Geometry: final body of the model. Coordinates: model frame, mm. A direction names the side the tool comes from. Round coordinates to 2 decimals unless told otherwise and drop trailing zeros. Loops run counter-clockwise (first coordinate to the right, second up) from the corner with the lowest first, then second, coordinate; pieces in that order, holes last. Notation, with made-up numbers: M -37.5,74 L -0.5,74 A12 cw -0.5,93 Z; hole C 0.25,87.5 d10. An arc over 180 degrees is marked long. Return JSON: item names as keys, results as strings.
from build123d import *

# Parameters (mm, degrees)
SKETCH1_R               = 6.35
BASE_BODY_DEPTH         = 10
SKETCH2_R               = 2.1
SHAFT_BEARING_CUT_DEPTH = 11
SKETCH3_OUTSIDE_W       = 18.812
SKETCH3_OUTSIDE_H       = 18.812
SKETCH3_OUTSIDE_R       = 4.1
LATHE_CUT_DEPTH         = 7.3


with BuildPart() as part:
    # Sketch1 → base_body (new body)
    with BuildSketch(Plane(origin=(0, 0, 0), x_dir=(1, 0, 0), z_dir=(0, 1, 0))):
        Circle(SKETCH1_R)
    extrude(amount=BASE_BODY_DEPTH)

    # Sketch2 → shaft_bearing_cut (cut, through all)
    with BuildSketch(Plane(origin=(0, 10, 0), x_dir=(1, 0, 0), z_dir=(0, 1, 0))):
        Circle(SKETCH2_R)
    extrude(amount=-SHAFT_BEARING_CUT_DEPTH, mode=Mode.SUBTRACT)

    # Sketch3 outside → lathe_cut (cut)
    with BuildSketch(Plane(origin=(0, 10, 0), x_dir=(1, 0, 0), z_dir=(0, 1, 0))):
        Rectangle(SKETCH3_OUTSIDE_W, SKETCH3_OUTSIDE_H)
        Circle(SKETCH3_OUTSIDE_R, mode=Mode.SUBTRACT)
    extrude(amount=-LATHE_CUT_DEPTH, mode=Mode.SUBTRACT)


solid = part.part
Q1. Section query D-D (x = -2.5). Output: boundary loops of the cut face in (y, z), plus the area to 3 significant figures.
Determined:
{"outline": "M 0,-5.84 L 2.7,-5.84 L 2.7,-3.25 L 10,-3.25 L 10,3.25 L 2.7,3.25 L 2.7,5.84 L 0,5.84 Z", "area": "79.0 mm^2"}
Q2. Section query B-B (z = 0). Output: boundary loops of the cut face in (x, y).
Determined:
{"outline": "M -6.35,0 L -2.1,0 L -2.1,10 L -4.1,10 L -4.1,2.7 L -6.35,2.7 Z; M 2.1,0 L 6.35,0 L 6.35,2.7 L 4.1,2.7 L 4.1,10 L 2.1,10 Z"}
Q3. Section query A-A (x = 0). Output: boundary loops of the cut face in (y, z).
Determined:
{"outline": "M 0,-6.35 L 2.7,-6.35 L 2.7,-4.1 L 10,-4.1 L 10,-2.1 L 0,-2.1 Z; M 0,2.1 L 10,2.1 L 10,4.1 L 2.7,4.1 L 2.7,6.35 L 0,6.35 Z"}
Q4. Material intervals for L1, parallel to X at y = 3.5, z = 0; L2, parallel to Y at x = 1, z = -4.25, sorted ascending.
Determined:
{"L1": "x = -4.1 to -2.1, 2.1 to 4.1", "L2": "y = 0 to 2.7"}
Q5. Reachability of faces 1 (the flat face through (1.3, 2.7, 4.1)), 2 (the flat face through (-2, 0, -2)) from +Z, -Z, +X, -X, +Y, -Y: full face, straight path, thin tool, end or side. Return the list, or none.
Determined:
{"face 1": "+Y", "face 2": "+Z, -Z, +X, -X, -Y"}
Q6. Pin query (flat end, axial travel): pin 1 (5 mm diameter, centred on x = 2.5, y = 5.5, fed in from -Z); pin 2 (1 mm diameter, centred on x = -2.5, z = 1, fed in from -Y); pin 3 (6 mm diameter, centred on x = -4.5, y = 3.5, fed in from -Z); pin 4 (6 mm diameter, centred on x = -4, y = 7.5, fed in from -Z). Return the tip coordinate at first contact, or that it passes through.
Determined:
{"pin 1": "stops at z = -4.1", "pin 2": "stops at y = 0", "pin 3": "stops at z = -6.14", "pin 4": "stops at z = -3.98"}
Q7. Section query C-C (y = 1.25). Output: boundary loops of the cut face in (x, z), plus the area to 3 significant figures.
Determined:
{"outline": "C 0,0 d12.7; hole C 0,0 d4.2", "area": "113 mm^2"}
Q8. Pull-direction query (Z, two-part tool) for faces 3 (the cylindrical face through (-0.534, 6.401, -4.065)), 4 (the flat face through (2, 10, 2)), 5 (the cylindrical face through (2.003, 5.07, -0.631)); classes: pulls with the +Z half, pulls with the -Z half, needs draft (parallel to the pull), parting line crosses it, or undercut.
Determined:
{"face 3": "parting line crosses it", "face 4": "needs draft", "face 5": "undercut"}
